Check sheet for the modelled part. Datum: model origin and axes. Units: mm. Give positions to 0.01 mm unless a question says otherwise; leave off trailing zeros. Order: outer loops, then holes, each group sorted by start corner. A loop starts at its lowest first (then second) coordinate and runs counter-clockwise, first axis right, second up. Notation, with made-up numbers: (63, 21.25) - (79, 21.25) arc R27 ccw to (79, 43.25) - close; hole circle Ø3 at (-31.75, 43.5). An arc over 180 degrees is marked (long way). Answer in a Markdown table with one row per item.
from build123d import *

# Parameters (mm, degrees)
SKETCH_1_R      = 2
SKETCH_1_R_2    = 10
SKETCH_1_R_3    = 4
EXTRUDE_1_DEPTH = 3


with BuildPart() as part:
    # 草图1 → 凸台-拉伸1 (new body)
    with BuildSketch(Plane(origin=(0, 0, 0), x_dir=(1, 0, 0), z_dir=(0, 1, 0))):
        with BuildLine():
            Line((-18.915, 88.196307868), (68.915, 88.196307868))
            ThreePointArc((68.915, 88.196307868), (75.986067812, 85.26737568), (78.915, 78.196307868))
            Line((78.915, 78.196307868), (78.915, -77.463692132))
            ThreePointArc((78.915, -77.463692132), (75.986067812, -84.534759944), (68.915, -87.463692132))
            Line((68.915, -87.463692132), (-18.915, -87.463692132))
            ThreePointArc((-18.915, -87.463692132), (-25.986067812, -84.534759944), (-28.915, -77.463692132))
            Line((-28.915, -77.463692132), (-28.915, 78.196307868))
            ThreePointArc((-28.915, 78.196307868), (-25.986067812, 85.26737568), (-18.915, 88.196307868))
        make_face()
        with Locations(Location((72.465, 81.936307868, 0), (0, 0, 270))):
            Circle(SKETCH_1_R, mode=Mode.SUBTRACT)
        with Locations(Location((72.465, -81.936307868, 0), (0, 0, 270))):
            Circle(SKETCH_1_R, mode=Mode.SUBTRACT)
        with Locations(Location((-22.465, -81.936307868, 0), (0, 0, 270))):
            Circle(SKETCH_1_R, mode=Mode.SUBTRACT)
        with Locations(Location((-22.465, 81.936307868, 0), (0, 0, 270))):
            Circle(SKETCH_1_R, mode=Mode.SUBTRACT)
        with Locations(Location((25, 40, 0), (0, 0, 270))):
            Circle(SKETCH_1_R_2, mode=Mode.SUBTRACT)
        with Locations(Location((11.26703509, 54, 0), (0, 0, 270))):
            Circle(SKETCH_1_R, mode=Mode.SUBTRACT)
        with Locations(Location((38.73296491, 54, 0), (0, 0, 270))):
            Circle(SKETCH_1_R, mode=Mode.SUBTRACT)
        with Locations(Location((38.73296491, 26, 0), (0, 0, 270))):
            Circle(SKETCH_1_R, mode=Mode.SUBTRACT)
        with Locations(Location((11.26703509, 26, 0), (0, 0, 270))):
            Circle(SKETCH_1_R, mode=Mode.SUBTRACT)
        with Locations(Location((11.26703509, -26, 0), (0, 0, 270))):
            Circle(SKETCH_1_R, mode=Mode.SUBTRACT)
        with Locations(Location((11.26703509, -54, 0), (0, 0, 270))):
            Circle(SKETCH_1_R, mode=Mode.SUBTRACT)
        with Locations(Location((25, -40, 0), (0, 0, 270))):
            Circle(SKETCH_1_R_2, mode=Mode.SUBTRACT)
        with Locations(Location((38.73296491, -26, 0), (0, 0, 270))):
            Circle(SKETCH_1_R, mode=Mode.SUBTRACT)
        with Locations(Location((38.73296491, -54, 0), (0, 0, 270))):
            Circle(SKETCH_1_R, mode=Mode.SUBTRACT)
        with Locations(Location((64.051731017, -0.006153743, 0), (0, 0, 270))):
            Circle(SKETCH_1_R, mode=Mode.SUBTRACT)
        with Locations(Location((-3.064799971, -0.006153743, 0), (0, 0, 270))):
            Circle(SKETCH_1_R_3, mode=Mode.SUBTRACT)
        with Locations(Location((-13.600868083, -0.006153743, 0), (0, 0, 270))):
            Circle(SKETCH_1_R, mode=Mode.SUBTRACT)
    extrude(amount=EXTRUDE_1_DEPTH)


solid = part.part
(1) Cross-section at B-B, the plane z = -48. Record the cut outline in (x, y) (3 decimals), then the cut area to 3 significant figures.
Geometry says:
| item | result |
|---|---|
| outline | (-28.915, 0) - (19, 0) - (19, 3) - (-28.915, 3) - close; (31, 0) - (78.915, 0) - (78.915, 3) - (31, 3) - close |
| area | 287 mm² |
(2) Mould release check, pull along X, two halves, no side actions. Record for faces 1 (the flat face through (26, 0, -2)), 2 (the cylindrical face through (-26.06, 1.48, -85.19)), 3 (the cylindrical face through (71.7, 1.48, -80.09)): pulls with the +X half, pulls with the -X half, needs draft (parallel to the pull), parting line crosses it, or undercut.
Geometry says:
| item | result |
|---|---|
| face 1 | needs draft |
| face 2 | pulls with the -X half |
| face 3 | undercut |
(3) Cross-section at A-A, the plane x = 25. Record the cut outline in (y, z), then the cut area to 3 significant figures.
Geometry says:
| item | result |
|---|---|
| outline | (0, -88.2) - (3, -88.2) - (3, -50) - (0, -50) - close; (0, -30) - (3, -30) - (3, 30) - (0, 30) - close; (0, 50) - (3, 50) - (3, 87.46) - (0, 87.46) - close |
| area | 407 mm² |
(4) Cross-section at C-C, the plane z = 54. Record the cut outline in (x, y) (3 decimals), then the cut area to 3 significant figures.
Geometry says:
| item | result |
|---|---|
| outline | (-28.915, 0) - (9.267, 0) - (9.267, 3) - (-28.915, 3) - close; (13.267, 0) - (36.733, 0) - (36.733, 3) - (13.267, 3) - close; (40.733, 0) - (78.915, 0) - (78.915, 3) - (40.733, 3) - close |
| area | 299 mm² |
(5) Thickness scan on L1, parallel to Z at x = 11.5, y = 2.3; L2, parallel to X at y = 1.4, z = 26 (3 decimals); L3, parallel to X at y = 1.9, z = 52.5 (3 decimals). Record the ranges inside material, lowest first.
Geometry says:
| item | result |
|---|---|
| L1 | -88.2 to -55.99, -52.01 to -27.99, -24.01 to 24.01, 27.99 to 52.01, 55.99 to 87.46 |
| L2 | -28.915 to 9.267, 13.267 to 36.733, 40.733 to 78.915 |
| L3 | -28.915 to 9.944, 12.59 to 37.41, 40.056 to 78.915 |
(6) Cross-section at D-D, the plane y = 1.7. Give the number of separate pieces and of enclosed holes in the cut face, then the cut area to 3 significant figures.
Geometry says:
| item | result |
|---|---|
| separate pieces | 1 |
| enclosed holes | 17 |
| area | 18,000 mm² |
